Check sheet for the modelled part. Datum: model origin and axes. Units: mm. Face numbers are marked on the shaded views. A direction names the side the tool comes from. Round coordinates to 2 decimals unless told otherwise and drop trailing zeros. Loops run counter-clockwise (first coordinate to the right, second up) from the corner with the lowest first, then second, coordinate; pieces in that order, holes last. Notation, with made-up numbers: (89.5, -10.75) - (123.5, -10.75) arc R22 cw to (123.5, 19.25) - close; hole circle Ø1 at (6.5, -30.5). An arc over 180 degrees is marked (long way). Put each result on its own line as item: value.
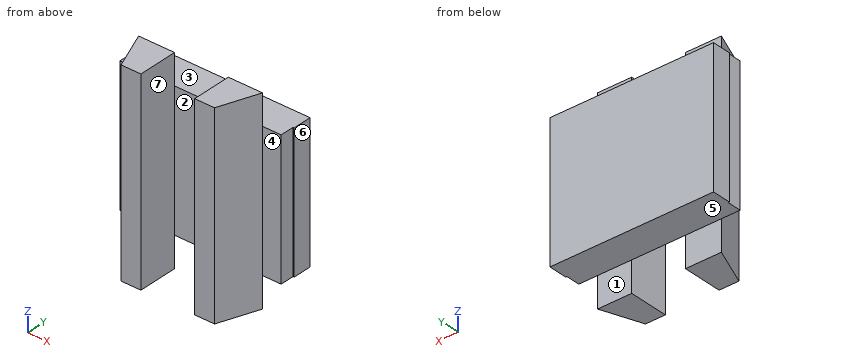
```python
from build123d import *

# Parameters (mm, degrees)
SKETCH_1_W           = 70
SKETCH_1_H           = 8
EXTRUDE_1_DEPTH      = 58
SKETCH_2_W           = 69
SKETCH_2_H           = 58
EXTRUDE_2_DEPTH      = 6
EXTRUDE_3_DEPTH      = 71
EXTRUDE_3_DEPTH_BACK = 13
CUT_EXTRUDE_2_REACH  = 103.107
SKETCH_6_W           = 23
SKETCH_6_H           = 16.995926687


with BuildPart() as part:
    # 草图1 → 凸台-拉伸1 (new body)
    with BuildSketch(Plane.XY):
        with Locations((16.857142857, 5.142857143)):
            Rectangle(SKETCH_1_W, SKETCH_1_H)
    extrude(amount=EXTRUDE_1_DEPTH)

    # 草图2 → 凸台-拉伸2 (add)
    with BuildSketch(Plane.XZ.offset(-1.142857143)):
        with Locations((16.857142857, 29)):
            Rectangle(SKETCH_2_W, SKETCH_2_H)
    extrude(amount=EXTRUDE_2_DEPTH)

    # 草图4 → 凸台-拉伸3 (add, two sides: drawn at the far end of the back side and taken through both)
    with BuildSketch(Plane.XY.offset(-EXTRUDE_3_DEPTH_BACK)):
        Polygon((-9.642857143, -4.857142857), (43.357142857, -4.857142857), (37.223942971, -21.853069544), (-2.776057029, -21.853069544), align=None)
    extrude(amount=EXTRUDE_3_DEPTH + EXTRUDE_3_DEPTH_BACK)

    # 草图6 → 切除-拉伸2 (cut, up to next)
    with BuildSketch(Plane.XY.offset(71), mode=Mode.PRIVATE) as cut_extrude_2_sk1:
        with Locations((17.223942971, -13.3551062)):
            Rectangle(SKETCH_6_W, SKETCH_6_H)
    cut_extrude_2_tool1 = extrude(cut_extrude_2_sk1.sketch, amount=-CUT_EXTRUDE_2_REACH, mode=Mode.PRIVATE) & part.part
    add(cut_extrude_2_tool1.solids().sort_by_distance((17.223943, -13.355106, 71))[0], mode=Mode.SUBTRACT)


solid = part.part
```
Item 1: Release check for a two-part mould opening along X. For the marked faces 5, 6 and 7 record: +X half, -X half, draft (parallel to the pull), parting line (faces both ways), or undercut.
Filled sheet:
face 5: draft
face 6: +X half
face 7: undercut
Item 2: Go/stop test with flat-tipped pins: pin 1 (5 mm diameter, centred on y = -2, z = 18.5, fed in from -X); pin 2 (11 mm diameter, centred on x = 27, y = 3.5, fed in from -Z); pin 3 (6.5 mm diameter, centred on x = 1, z = 66.5, fed in from +Y); pin 4 (1.5 mm diameter, centred on x = 7.5, z = -3, fed in from -Y). Record where each tip stops, or that it passes through.
Filled sheet:
pin 1: x = -17.64
pin 2: z = 0
pin 3: y = -4.86
pin 4: through
Item 3: Section check D-D on y = -7. Enter the section's corners in (x, z), then the cut area to 3 significant figures.
Filled sheet:
outline: (-8.78, -13) - (5.72, -13) - (5.72, 71) - (-8.78, 71) - close; (28.72, -13) - (42.58, -13) - (42.58, 71) - (28.72, 71) - close
area: 2,380 mm²
Item 4: Thickness scan on line 1 (X direction, y = -11.5, z = -3); line 2 (X direction, y = -12, z = 10); line 3 (Y direction, x = 25, z = 29.5). Record the ranges inside material, lowest first. Write a range as from..to.
Filled sheet:
line 1: -6.96..5.72, 28.72..40.96
line 2: -6.76..5.72, 28.72..40.78
line 3: -4.86..9.14
Item 5: Section check A-A on y = -19. Enter the section's corners in (x, z), then the cut area to 3 significant figures.
Filled sheet:
outline: (-3.93, -13) - (5.72, -13) - (5.72, 71) - (-3.93, 71) - close; (28.72, -13) - (38.25, -13) - (38.25, 71) - (28.72, 71) - close
area: 1,610 mm²
Item 6: Section check B-B on z = 46. Enter the section's corners in (x, y).
Filled sheet:
outline: (-18.14, 1.14) - (-17.64, 1.14) - (-17.64, -4.86) - (-9.64, -4.86) - (-2.78, -21.85) - (5.72, -21.85) - (5.72, -4.86) - (28.72, -4.86) - (28.72, -21.85) - (37.22, -21.85) - (43.36, -4.86) - (51.36, -4.86) - (51.36, 1.14) - (51.86, 1.14) - (51.86, 9.14) - (-18.14, 9.14) - close
Item 7: Section check C-C on x = -1.5. Enter the section's corners in (y, z), then the cut area to 3 significant figures.
Filled sheet:
outline: (-21.85, -13) - (-4.86, -13) - (-4.86, 0) - (9.14, 0) - (9.14, 58) - (-4.86, 58) - (-4.86, 71) - (-21.85, 71) - close
area: 2,240 mm²
Item 8: Tool access check on the marked faces 1, 2, 3 and 4. Record the directions out of +Z, -Z, +X, -X, +Y, -Y that give a thin tool (end or side, any length) a straight path to the whole face; none if there is none.
Filled sheet:
face 1: -Z, +X, -X, +Y
face 2: +Z, -Z, -Y
face 3: +Z, +X, -X, +Y
face 4: +Z, -Z, +X, -Y
